Verification items for the finished model (mm, model axes). Face numbers are marked on the shaded views. A direction names the side the tool comes from. Round coordinates to 2 decimals unless told otherwise and drop trailing zeros. Order: outer loops, then holes, each group sorted by start corner. A loop starts at its lowest first (then second) coordinate and runs counter-clockwise, first axis right, second up. Notation, with made-up numbers: M -10,-17 L 0,-17 A20 cw 0,-7 Z; hole C 7.25,14.5 d1. An arc over 180 degrees is marked long. Use one line per item in the form item = value. Start each with the question number.
Item 1: Go/stop test with flat-tipped pins: pin 1 Ø6 at (x, y) = (19, -4) entering from +Z; pin 2 Ø1 at (y, z) = (-21, 5.5) entering from -X; pin 3 Ø15 at (y, z) = (-16.5, -9) entering from -X (3 decimals); pin 4 Ø4 at (x, z) = (-27, -16) entering from -Y. Record where each tip stops, or that it passes through.
Item 2: Cross-section at B-B on z = -2. Enter the section's corners in (x, y) (3 decimals), then the cut area to 3 significant figures.
Item 3: Tool access check on the marked faces 5, 6 and 7. Record the directions out of +Z, -Z, +X, -X, +Y, -Y that give a thin tool (end or side, any length) a straight path to the whole face; none if there is none.
Item 4: Cross-section at A-A on x = 0. Enter the section's corners in (y, z) (3 decimals).
Item 5: Cross-section at D-D on z = -12. Enter the section's corners in (x, y) (3 decimals).
Item 6: Cross-section at C-C on y = -9. Enter the section's corners in (x, z) (3 decimals), then the cut area to 3 significant figures.
Item 7: Thickness scan on probe 1 along Z at (x, y) = (0, -7) (3 decimals); probe 2 along X at (y, z) = (-21, -14.5) (3 decimals); probe 3 along Y at (x, z) = (13.5, -19.5). Record the ranges inside material, lowest first. Write a range as [from, to].
Item 8: Release check for a two-part mould opening along Z. For the marked faces 1, 2, 3 and 4 record: +Z half, -Z half, draft (parallel to the pull), parting line (faces both ways), or undercut.
from build123d import *

# Parameters (mm, degrees)
F0_R     = 9.525
F1_DEPTH = 25.4
F2_R     = 2.54


with BuildPart() as f1:
    # F0 (on Front) → F1 (new body)
    with BuildSketch(Plane.XZ):
        with BuildLine():
            Line((15.875, -19.05), (15.875, 0))
            ThreePointArc((15.875, 0), (0, 15.875), (-15.875, 0))
            Line((-15.875, 0), (-15.875, -19.05))
            Line((-15.875, -19.05), (-38.1, -19.05))
            Line((-38.1, -19.05), (-38.1, -25.4))
            Line((-38.1, -25.4), (0, -25.4))
            Line((0, -25.4), (38.1, -25.4))
            Line((38.1, -25.4), (38.1, -19.05))
            Line((38.1, -19.05), (15.875, -19.05))
        make_face()
        Circle(F0_R, mode=Mode.SUBTRACT)
    extrude(amount=F1_DEPTH)

    # F2
    f2_edges = [f1.edges().sort_by_distance(p)[0] for p in [
        (0, -25.4, 15.875),
        (0, 0, 15.875),
        (-15.875, -25.4, -9.525),
        (15.875, -25.4, -9.525),
        (26.9875, -25.4, -19.05),
        (-26.9875, -25.4, -19.05),
        (-38.1, -12.7, -19.05),
        (-26.9875, 0, -19.05),
        (-15.875, 0, -9.525),
        (15.875, 0, -9.525),
        (26.9875, 0, -19.05),
        (38.1, -12.7, -19.05),
        (-38.1, -25.4, -22.225),
        (-38.1, 0, -22.225),
        (38.1, 0, -22.225),
        (38.1, -25.4, -22.225),
    ]]
    fillet(f2_edges, radius=F2_R)


solid = f1.part
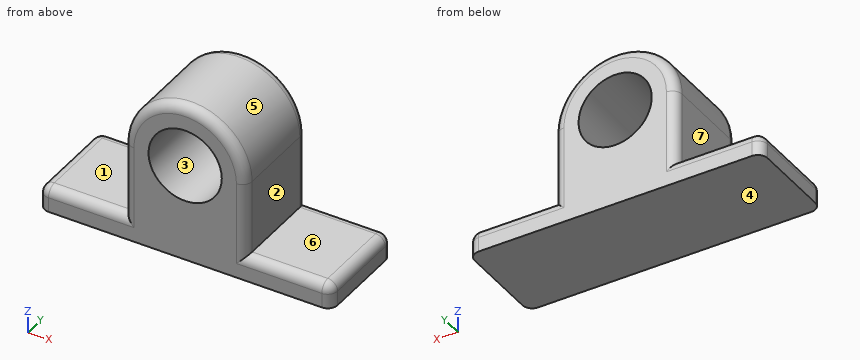
Output values:
q1.pin_1 = -19.05
q1.pin_2 = -15.07
q1.pin_3 = -15.875
q1.pin_4 = through
q2.outline = M -15.875,-22.86 A2.54 ccw -13.335,-25.4 L -9.313,-25.4 L -9.313,0 L -13.335,0 A2.54 ccw -15.875,-2.54 Z; M 9.313,-25.4 L 13.335,-25.4 A2.54 ccw 15.875,-22.86 L 15.875,-2.54 A2.54 ccw 13.335,0 L 9.313,0 Z
q2.area = 328 mm2
q3.face_5 = +Z, +Y, -Y
q3.face_6 = +Z, +X, +Y, -Y
q3.face_7 = +Z, -X, +Y, -Y
q4.outline = M -25.4,-25.4 L 0,-25.4 L 0,-9.525 L -25.4,-9.525 Z; M -25.4,9.525 L 0,9.525 L 0,13.335 A2.54 ccw -2.54,15.875 L -22.86,15.875 A2.54 ccw -25.4,13.335 Z
q5.outline = M -15.875,-22.86 A2.54 ccw -13.335,-25.4 L 13.335,-25.4 A2.54 ccw 15.875,-22.86 L 15.875,-2.54 A2.54 ccw 13.335,0 L -13.335,0 A2.54 ccw -15.875,-2.54 Z
q6.outline = M -38.1,-25.4 L 38.1,-25.4 L 38.1,-21.59 A2.54 ccw 35.56,-19.05 L 15.875,-19.05 L 15.875,0 A15.875 ccw -15.875,0 L -15.875,-19.05 L -35.56,-19.05 A2.54 ccw -38.1,-21.59 Z; hole C 0,0 d19.05
q6.area = 1,200 mm2
q7.probe_1 = [-25.4, -9.525], [9.525, 15.875]
q7.probe_2 = [-15.875, 15.875]
q7.probe_3 = [-25.39, -0.01]
q8.face_1 = +Z half
q8.face_2 = draft
q8.face_3 = undercut
q8.face_4 = -Z half
